Autodesk Inventor part; units mm, degrees
ref_plane "YZ Plane" through (0, 0, 0) normal (1, 0, 0) x (0, 1, 0)
ref_plane "XZ Plane" through (0, 0, 0) normal (0, 1, 0) x (-1, 0, 0)
ref_plane "XY Plane" through (0, 0, 0) normal (0, 0, 1) x (1, 0, 0)
sketch "Sketch1" plane through (0, 0, 0) normal (1, 0, 0) x (0, 1, 0)
  line L0 (0, 0) -> (179, 0)
  line L1 (179, 0) -> (179, -109)
  line L2 (179, -109) -> (0, -109)
  line L3 (0, -109) -> (0, 0)
  dimension "d0" = 179
  dimension "d1" = 109
extrude "Extrusion1" add sketch "Sketch1" along normal blind 10
sketch "Sketch2" plane through (0, 179, 0) normal (0, 1, 0) x (1, 0, 0)
  point P0 (0, 0)
sketch "Sketch3" plane through (0, 179, 0) normal (0, 1, 0) x (1, 0, 0)
  line L0 (0, 109) -> (10, 101.9979)
  line L1 (10, 109) -> (10, 0)
  line L2 (0, 109) -> (0, 0)
  line L3 (0, 0) -> (10, 0)
  line L4 (0, 0) -> (10, 7.0021)
  dimension "d4" = 125
  dimension "d5" = 125
extrude "Extrusion2" cut sketch "Sketch3" against normal through all contours L4 L1 L3
sketch "Sketch4" plane through (0, 179, -109) normal (0, 1, 0) x (1, 0, 0)
  point P0 (0, -109)
sketch "Sketch5" plane through (0, 179, -109) normal (0, 1, 0) x (1, 0, 0)
  line L0 (0, -109) -> (0, 0)
  line L1 (10, 0) -> (10, -101.9979)
sketch "Sketch6" plane through (0, 179, -109) normal (0, 1, 0) x (1, 0, 0)
  line L0 (0, -109) -> (0, 0)
  line L1 (0, 0) -> (10, -7.0021)
  line L2 (10, 0) -> (10, -101.9979)
  line L3 (0, 0) -> (10, 0)
  line L4 (0, 0) -> (10, 0)
  line L5 (10, 0) -> (10, -7.0021)
  dimension "d8" = 125
extrude "Extrusion3" cut sketch "Sketch6" against normal through all
sketch "Sketch7" plane through (10, 0, 0) normal (1, 0, 0) x (0, 0, -1)
  point P0 (0, 0)
sketch "Sketch8" plane through (10, 0, 0) normal (1, 0, 0) x (0, 0, -1)
  line L0 (47.4589, 117) -> (60.4589, 117)
  line L1 (60.4589, 117) -> (60.4589, 75)
  line L2 (60.4589, 75) -> (47.4589, 75)
  line L3 (47.4589, 75) -> (47.4589, 117)
  line L4 (101.9979, 179) -> (7.0021, 179)
  point P0 (0, 0)
  dimension "d11" = 13
  dimension "d12" = 42
  dimension "d13" = 62
extrude "Extrusion4" cut sketch "Sketch8" against normal through all
sketch "Sketch9" plane through (0, 0, 0) normal (0.5736, 0, 0.8192) x (0.8192, 0, -0.5736)
  point P0 (0, 0)
sketch "Sketch10" plane through (0, 0, 0) normal (0.5736, 0, 0.8192) x (0.8192, 0, -0.5736)
  point P0 (0, 0)
sketch "Sketch11" plane through (0, 179, 0) normal (0, 1, 0) x (1, 0, 0)
  line L0 (0, 109) -> (0, 0)
  line L1 (0, 109) -> (0.5, 109)
  line L2 (0.5, 109) -> (0.5, 0)
  line L3 (0.5, 0) -> (0, 0)
  line L4 (0, 0) -> (0, 109)
  dimension "d16" = 0.5
extrude "Extrusion5" cut sketch "Sketch11" against normal through all
Input: part model. Units: mm. Frame: model coordinates. A direction names the side the tool comes from. Give positions to 0.01 mm unless a question says otherwise; leave off trailing zeros. Write each loop counter-clockwise with the first axis right and the second up, starting at its lowest first coordinate (ties: lowest second). Pieces come first, ordered by that corner, then holes.
Q1. Section A-A, the plane y = 95.5. Output: boundary loops of the cut face in (x, z), plus the area to 3 significant figures.
Q2. Material intervals for probe 1 along Y at (x, z) = (2.5, -57); probe 2 along Z at (x, y) = (4.25, 90); probe 3 along Z at (x, y) = (9, 76.5), sorted ascending.
Q3. Section B-B, the plane z = -50. Output: boundary loops of the cut face in (x, y).
Q4. Section D-D, the plane y = 57.5. Output: boundary loops of the cut face in (x, z).
Q5. Set-up query: faces 1 (the face through (5, 96, -60.459)), 2 (the face through (0.5, 91, -43)). Return all of +Z, -Z, +X, -X, +Y, -Y with unobstructed straight access to the full face (end or side cutting, diameter ignored); none if empty.
Q6. Section C-C, the plane x = 3.5. Output: boundary loops of the cut face in (y, z).
Q7. Pull-direction query (Y, two-part tool) for faces 3 (the face through (5.184, 90.753, -105.37)), 4 (the face through (5, 96, -47.459)), 5 (the face through (5, 179, -54)); classes: pulls with the +Y half, pulls with the -Y half, needs draft (parallel to the pull), parting line crosses it, or undercut.
Q8. First-contact query: P1, Ø3, axis at x = 3, z = -55.5, coming from the -Y side; P2, Ø3, axis at x = 1.5, y = 74.5, coming from the -Z side; P3, Ø1, axis at x = 2, y = 114, coming from the +Z side; P4, Ø3, axis at x = 7, y = 101, coming from the -Z side. Flat tips, straight axial feed; report the tip coordinate or a pass-through.
Filled in:
1. outline: (0.5, -108.65) - (10, -102) - (10, -60.46) - (0.5, -60.46) - close; (0.5, -47.46) - (10, -47.46) - (10, -7) - (0.5, -0.35) - close
1. area: 842 mm2
2. probe 1: y = 0 to 75, 117 to 179
2. probe 2: z = -106.02 to -60.46, -47.46 to -2.98
2. probe 3: z = -102.7 to -60.46, -47.46 to -6.3
3. outline: (0.5, 0) - (10, 0) - (10, 75) - (0.5, 75) - close; (0.5, 117) - (10, 117) - (10, 179) - (0.5, 179) - close
4. outline: (0.5, -108.65) - (10, -102) - (10, -7) - (0.5, -0.35) - close
5. face 1: +X, -X
5. face 2: +Z, -Z, -X, +Y, -Y
6. outline: (0, -106.55) - (179, -106.55) - (179, -2.45) - (0, -2.45) - close; hole (75, -60.46) - (117, -60.46) - (117, -47.46) - (75, -47.46) - close
7. face 3: needs draft
7. face 4: undercut
7. face 5: pulls with the +Y half
8. P1: stops at y = 0
8. P2: stops at z = -108.65
8. P3: stops at z = -1.05
8. P4: stops at z = -105.15
